from build123d import *

# Parameters (mm, degrees)
ESBO_O1_R                  = 14.5
RESSALTO_EXTRUS_O1_DEPTH   = 30
ESBO_O3_R                  = 7.5
CORTE_EXTRUS_O3_DEPTH      = 17
FILETE1_R                  = 7
FILETE2_R                  = 2
CORTE_EXTRUS_O1_DEPTH      = 36.994872408
CORTE_EXTRUS_O1_DEPTH_BACK = 36.994872408
ESBO_O2_R                  = 2
ESBO_O1_3_R                = 2
CORTE_EXTRUS_O2_DEPTH      = 10


with BuildPart() as part:
    # Esboço1 → Ressalto-extrusão1 (new body)
    with BuildSketch(Plane(origin=(0, 0, 0), x_dir=(1, 0, 0), z_dir=(0, 1, 0))):
        with Locations(Location((0, 0, 0), (0, 0, 270))):
            Circle(ESBO_O1_R)
    extrude(amount=RESSALTO_EXTRUS_O1_DEPTH)

    # Esboço3 → Corte-extrusão3 (cut)
    with BuildSketch(Plane(origin=(0, 30, 0), x_dir=(1, 0, 0), z_dir=(0, 1, 0))):
        with Locations(Location((0, 0, 0), (0, 0, 270))):
            Circle(ESBO_O3_R)
    extrude(amount=-CORTE_EXTRUS_O3_DEPTH, mode=Mode.SUBTRACT)

    # Filete1
    filete1_edges = [part.edges().sort_by_distance(p)[0] for p in [
        (0, 13, -7.5),
        (0, 30, -7.5),
    ]]
    fillet(filete1_edges, radius=FILETE1_R - 0.0001)  # a hair under: the kernel refuses the full size

    # Filete2
    filete2_edges = [part.edges().sort_by_distance(p)[0] for p in [
        (0, 30, -14.5),
    ]]
    fillet(filete2_edges, radius=FILETE2_R)

    # Esboço2 → Corte-extrusão1 (cut, two sides: drawn at the far end of the back side and taken through both)
    with BuildSketch(Plane(origin=(0, 0, 0), x_dir=(0, 0, -1), z_dir=(1, 0, 0)).offset(-CORTE_EXTRUS_O1_DEPTH_BACK)):
        with Locations((0, 15)):
            Circle(ESBO_O2_R)
    extrude(amount=CORTE_EXTRUS_O1_DEPTH + CORTE_EXTRUS_O1_DEPTH_BACK, mode=Mode.SUBTRACT)

    # Esboço1<3> → Corte-extrusão2 (cut)
    with BuildSketch(Plane(origin=(0, 0, 0), x_dir=(1, 0, 0), z_dir=(0, 1, 0))):
        with Locations(Location((-7.25, 0, 0), (0, 0, 270))):
            Circle(ESBO_O1_3_R)
        with BuildLine():
            ThreePointArc((3.175, 0), (2.24506403, 2.24506403), (0, 3.175))
            Line((0, 3.175), (0, -3.175))
            ThreePointArc((0, -3.175), (2.24506403, -2.24506403), (3.175, 0))
        make_face()
        with BuildLine():
            Line((0, -3.175), (0, 3.175))
            ThreePointArc((0, 3.175), (-3.175, 0), (0, -3.175))
        make_face()
        with Locations(Location((7.25, 0, 0), (0, 0, 270))):
            Circle(ESBO_O1_3_R)
    extrude(amount=CORTE_EXTRUS_O2_DEPTH, mode=Mode.SUBTRACT)


solid = part.part
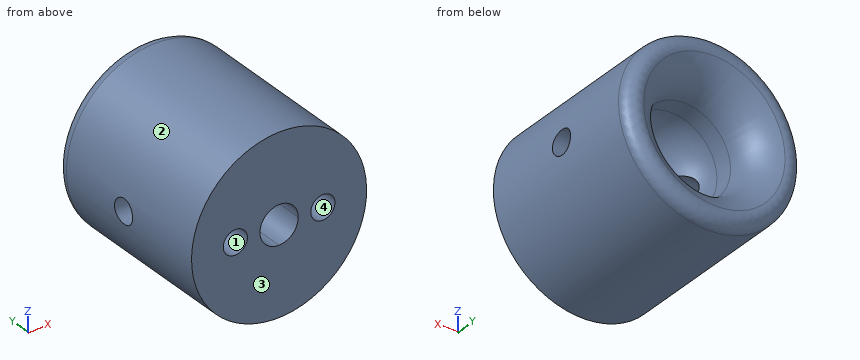
Can you work these out from the model? Positions are in its coordinate system, mm. Face numbers are marked on the shaded views. Round coordinates to 2 decimals unless told otherwise and drop trailing zeros. Use a Markdown table: item, result.
Item 1: For pin 1 Ø5 at (y, z) = (3, 10) entering from -X; pin 2 Ø2 at (x, z) = (-7, 0) entering from -Y; pin 3 Ø3 at (x, z) = (-7.25, 0) entering from +Y, each with a flat end and sliding along its axis, tell me the tip position at first contact or that it passes through.
Found:
| item | result |
|---|---|
| pin 1 | stops at x = -12.41 |
| pin 2 | stops at y = 10 |
| pin 3 | stops at y = 26.99 |
Item 2: If I drill on line 1 along X through (y, z) = (21.55, 0); line 2 along Y through (x, z) = (-4.5, 0); line 3 along Z through (x, y) = (-6, 4.5), over which ranges is the centre line in solid material (lowest first)? Write a range as [from, to].
Found:
| item | result |
|---|---|
| line 1 | x = [-14.5, -7.5], [7.5, 14.5] |
| line 2 | y = [0, 13] |
| line 3 | z = [-13.2, -1.56], [1.56, 13.2] |
Item 3: We'd pull the mould along Z, two halves only. Please class the marked faces 1, 2, 3 and 4: released by +Z, released by -Z, zero draft, split by the parting line, or undercut.
Found:
| item | result |
|---|---|
| face 1 | undercut |
| face 2 | split by the parting line |
| face 3 | zero draft |
| face 4 | undercut |
